For this review, take the finished solid that the model builds, in its own axes (mm). A direction names the side the tool comes from. Coordinates: 2 decimals unless noted, no trailing zeros. Loops run counter-clockwise (first coordinate to the right, second up) from the corner with the lowest first, then second, coordinate; pieces in that order, holes last. Notation, with made-up numbers: (25.25, 1.25) - (56.25, 1.25) arc R22 cw to (56.25, 29.25) - close; hole circle Ø9 at (-19.75, 85.5). An arc over 180 degrees is marked (long way). Answer as a JSON object with one key per item and string values. Group by question number.
Item 1: We need section A-A (y = 1.5). Give the boundary of the cut face in (x, z).
Item 2: We need section C-C (z = -7.5). Give the boundary of the cut face in (x, y), then the cut area to 3 significant figures.
Item 3: Clearance check with flat-ended pins moving along their axes: pin 1 (0.5 mm diameter, centred on y = 1, z = 2.5, fed in from -X); pin 2 (6 mm diameter, centred on x = 11.5, z = -9, fed in from -Y); pin 3 (3.5 mm diameter, centred on x = 10.74, z = 2, fed in from +Y); pin 4 (10 mm diameter, centred on y = 2.5, z = -9.5, fed in from +X). State where each tip first meets the part, or that it passes through.
Item 4: Mouldability with a two-part tool opening along Z and no side actions: class faces 6 (the flat face through (10, 8, -8)), 7 (the flat face through (3, 15, -14)), 8 (the cylindrical face through (6.35, 13.01, -8.08)) as released by +Z, released by -Z, zero draft, split by the parting line, or undercut.
Item 5: Tool access review of faces 1 (the cylindrical face through (1.77, 24.64, -13.1)), 2 (the flat face through (12.8, 2.5, 4.5)), 3 (the flat face through (9, 2.4, 3)), 4 (the flat face through (9, -1, -15)), 5 (the flat face through (3.5, 23, -8)): name each direction out of +Z, -Z, +X, -X, +Y, -Y from which nothing blocks a thin tool from reaching the whole face with its end or side.
Item 6: To check wall thickness, follow line 1 (Z direction, x = 10.74, y = -0.3); line 2 (Z direction, x = 10.74, y = 6.5); line 3 (X direction, y = 1, z = 2). State the ranges of each line that lie inside material, in increasing order.
Item 7: We need section B-B (y = 5.75). Give the boundary of the cut face in (x, z), then the cut area to 3 significant figures.
Item 8: We need section D-D (x = 2). Give the boundary of the cut face in (y, z), then the cut area to 3 significant figures.
from build123d import *

# Parameters (mm, degrees)
SALIENTE_EXTRUIR1_DEPTH = 10
CORTAR_EXTRUIR1_DEPTH   = 8
CROQUIS3_W              = 9
CROQUIS3_H              = 2.5
SALIENTE_EXTRUIR2_DEPTH = 5
CROQUIS4_R              = 1.5499999999999994
CORTAR_EXTRUIR2_DEPTH   = 2.5
REDONDEO1_R             = 2
CROQUIS5_R              = 2.9
CORTAR_EXTRUIR3_DEPTH   = 7.6
SALIENTE_EXTRUIR3_DEPTH = 15.5
REDONDEO2_R             = 10
REDONDEO3_R             = 3
CROQUIS8_R              = 1.5499999999999994
SALIENTE_EXTRUIR5_DEPTH = 1
CROQUIS9_W              = 5
CROQUIS9_H              = 1.700000000000001
CORTAR_EXTRUIR4_DEPTH   = 36.46565245064583


with BuildPart() as part:
    # Croquis1 → Saliente-Extruir1 (new body)
    with BuildSketch(Plane(origin=(0, 0, 0), x_dir=(1, 0, 0), z_dir=(0, 1, 0))):
        Polygon((0, 0), (18.75, 0), (18.749999999999996, 16), (-3.47e-15, 16), align=None)
    extrude(amount=SALIENTE_EXTRUIR1_DEPTH)

    # Croquis2 → Cortar-Extruir1 (cut)
    with BuildSketch(Plane.XZ):
        Polygon((0, -1.7000000000000002), (18.749999999999993, -1.6999999999999997), (18.749999999999996, -14.3), (1.51e-15, -14.3), align=None)
    extrude(amount=-CORTAR_EXTRUIR1_DEPTH, mode=Mode.SUBTRACT)

    # Croquis3 → Saliente-Extruir2 (add)
    with BuildSketch(Plane.XY):
        with Locations((10.750000000000002, 1.25)):
            Rectangle(CROQUIS3_W, CROQUIS3_H)
    extrude(amount=SALIENTE_EXTRUIR2_DEPTH)

    # Croquis4 → Cortar-Extruir2 (cut)
    with BuildSketch(Plane(origin=(0, 2.5, 0), x_dir=(1, 0, 0), z_dir=(0, 1, 0))):
        with Locations(Location((10.74, -2, 0), (0, 0, 270))):
            Circle(CROQUIS4_R)
    extrude(amount=-CORTAR_EXTRUIR2_DEPTH, mode=Mode.SUBTRACT)

    # Redondeo1
    # the kernel refuses this fillet: 2 mm, written as the material it adds along each edge
    with BuildSketch(Plane(origin=(6.25, 2.5, 0), x_dir=(-1, 0, 0), z_dir=(0, -1, 0))) as redondeo1_piece_1:
        with BuildLine():
            CenterArc((REDONDEO1_R, -REDONDEO1_R), REDONDEO1_R, 90, 90)
            Line((0, -REDONDEO1_R), (0, 0))
            Line((0, 0), (REDONDEO1_R, 0))
        make_face()
    extrude(amount=2.5)
    with BuildSketch(Plane(origin=(15.25, 0, 0), x_dir=(1, 0, 0), z_dir=(0, 1, 0))) as redondeo1_piece_2:
        with BuildLine():
            CenterArc((REDONDEO1_R, -REDONDEO1_R), REDONDEO1_R, 90, 90)
            Line((0, -REDONDEO1_R), (0, 0))
            Line((0, 0), (REDONDEO1_R, 0))
        make_face()
    extrude(amount=2.5)
    with BuildSketch(Plane(origin=(15.25, 2.5, 0), x_dir=(0, 1, 0), z_dir=(-1, 0, 0))) as redondeo1_piece_3_section:
        with BuildLine():
            CenterArc((REDONDEO1_R, -REDONDEO1_R), REDONDEO1_R, 90, 90)
            Line((0, -REDONDEO1_R), (0, 0))
            Line((0, 0), (REDONDEO1_R, 0))
        make_face()
    redondeo1_piece_3 = extrude(amount=9, mode=Mode.PRIVATE)
    redondeo1_piece_3 = redondeo1_piece_3 - Plane(origin=(10.74, 2.981912580650479, 2), x_dir=(-1.8e-16, 0, 1), z_dir=(0, 1, 0)) * Cylinder(1.5499999999999994, 26, mode=Mode.PRIVATE)
    add(redondeo1_piece_3)
    with BuildSketch(Plane(origin=(6.25, 7.5, 0), x_dir=(-1, 0, 0), z_dir=(0, -1, 0))) as redondeo1_piece_4a_section:
        with BuildLine():
            CenterArc((REDONDEO1_R, -REDONDEO1_R), REDONDEO1_R, 90, 90)
            Line((0, -REDONDEO1_R), (0, 0))
            Line((0, 0), (REDONDEO1_R, 0))
        make_face()
    redondeo1_piece_4a = extrude(amount=7.5, mode=Mode.PRIVATE)
    redondeo1_piece_4a = split(redondeo1_piece_4a, bisect_by=Plane(origin=(5.797209771466349, 2.5, 0.45279022853365075), z_dir=(0, 1, 0)), keep=Keep.TOP, mode=Mode.PRIVATE)
    with BuildSketch(Plane(origin=(15.25, 2.5, 0), x_dir=(0, 1, 0), z_dir=(-1, 0, 0))) as redondeo1_piece_4b_section:
        with BuildLine():
            CenterArc((REDONDEO1_R, -REDONDEO1_R), REDONDEO1_R, 90, 90)
            Line((0, -REDONDEO1_R), (0, 0))
            Line((0, 0), (REDONDEO1_R, 0))
        make_face()
    redondeo1_piece_4b = extrude(amount=14, mode=Mode.PRIVATE)
    redondeo1_piece_4b = split(redondeo1_piece_4b, bisect_by=Plane(origin=(6.25, 2.952790228533651, 0.45279022853365075), z_dir=(-1, 0, 0)), keep=Keep.TOP, mode=Mode.PRIVATE)
    redondeo1_piece_4 = redondeo1_piece_4a & redondeo1_piece_4b
    add(redondeo1_piece_4)
    with BuildSketch(Plane(origin=(20.25, 2.5, 0), x_dir=(0, 1, 0), z_dir=(-1, 0, 0))) as redondeo1_piece_5a_section:
        with BuildLine():
            CenterArc((REDONDEO1_R, -REDONDEO1_R), REDONDEO1_R, 90, 90)
            Line((0, -REDONDEO1_R), (0, 0))
            Line((0, 0), (REDONDEO1_R, 0))
        make_face()
    redondeo1_piece_5a = extrude(amount=14, mode=Mode.PRIVATE)
    redondeo1_piece_5a = split(redondeo1_piece_5a, bisect_by=Plane(origin=(18.75, 2.952790228533651, 0.45279022853365036), z_dir=(-1, 0, 2.2e-16)), keep=Keep.TOP, mode=Mode.PRIVATE)
    redondeo1_piece_5a = split(redondeo1_piece_5a, bisect_by=Plane(origin=(15.25, 2.952790228533651, 0.45279022853365075), z_dir=(1, 0, 0)), keep=Keep.TOP, mode=Mode.PRIVATE)
    with BuildSketch(Plane(origin=(15.25, 0, 0), x_dir=(1, 0, 0), z_dir=(0, 1, 0))) as redondeo1_piece_5b_section:
        with BuildLine():
            CenterArc((REDONDEO1_R, -REDONDEO1_R), REDONDEO1_R, 90, 90)
            Line((0, -REDONDEO1_R), (0, 0))
            Line((0, 0), (REDONDEO1_R, 0))
        make_face()
    redondeo1_piece_5b = extrude(amount=7.5, mode=Mode.PRIVATE)
    redondeo1_piece_5b = split(redondeo1_piece_5b, bisect_by=Plane(origin=(15.70279022853365, 2.5, 0.45279022853364964), z_dir=(0, 1, 0)), keep=Keep.TOP, mode=Mode.PRIVATE)
    redondeo1_piece_5 = redondeo1_piece_5a & redondeo1_piece_5b
    add(redondeo1_piece_5)
    # the kernel refuses this fillet: 2 mm, written as the material it takes off along each edge
    with BuildSketch(Plane(origin=(23.749999999999996, 10, -16), x_dir=(0, -1, 0), z_dir=(-1, 0, 0))) as redondeo1_2_piece_1:
        with BuildLine():
            CenterArc((REDONDEO1_R, REDONDEO1_R), REDONDEO1_R, 180, 90)
            Line((0, REDONDEO1_R), (0, 0))
            Line((0, 0), (REDONDEO1_R, 0))
        make_face()
    extrude(amount=28.75, mode=Mode.SUBTRACT)
    with BuildSketch(Plane(origin=(6.25, 7.5, 5), x_dir=(0, 0, -1), z_dir=(0, -1, 0))) as redondeo1_2_piece_2:
        with BuildLine():
            CenterArc((REDONDEO1_R, REDONDEO1_R), REDONDEO1_R, 180, 90)
            Line((0, REDONDEO1_R), (0, 0))
            Line((0, 0), (REDONDEO1_R, 0))
        make_face()
    extrude(amount=12.5, mode=Mode.SUBTRACT)
    with BuildSketch(Plane(origin=(15.25, -5, 5), x_dir=(0, 0, -1), z_dir=(0, 1, 0))) as redondeo1_2_piece_3:
        with BuildLine():
            CenterArc((REDONDEO1_R, REDONDEO1_R), REDONDEO1_R, 180, 90)
            Line((0, REDONDEO1_R), (0, 0))
            Line((0, 0), (REDONDEO1_R, 0))
        make_face()
    extrude(amount=12.5, mode=Mode.SUBTRACT)
    with BuildSketch(Plane(origin=(-5, 10, 0), x_dir=(0, -1, 0), z_dir=(1, 0, 0))) as redondeo1_2_piece_4:
        with BuildLine():
            CenterArc((REDONDEO1_R, REDONDEO1_R), REDONDEO1_R, 180, 90)
            Line((0, REDONDEO1_R), (0, 0))
            Line((0, 0), (REDONDEO1_R, 0))
        make_face()
    extrude(amount=28.75, mode=Mode.SUBTRACT)

    # Croquis5 → Cortar-Extruir3 (cut)
    with BuildSketch(Plane(origin=(0, 10, 0), x_dir=(1, 0, 0), z_dir=(0, 1, 0))):
        with Locations(Location((10.74, -2, 0), (0, 0, 270))):
            Circle(CROQUIS5_R)
    extrude(amount=-CORTAR_EXTRUIR3_DEPTH, mode=Mode.SUBTRACT)

    # Croquis6 → Saliente-Extruir3 (add)
    with BuildSketch(Plane(origin=(0, 10, 0), x_dir=(1, 0, 0), z_dir=(0, 1, 0))):
        Polygon((-3.04e-15, 14), (3.499999999999997, 14), (3.4999999999999982, 2), (-3.04e-15, 2), align=None)
    extrude(amount=SALIENTE_EXTRUIR3_DEPTH)

    # Redondeo2
    # the kernel refuses this fillet: 10 mm, written as the material it adds along each edge
    with BuildSketch(Plane(origin=(3.499999999999997, 10, -14), x_dir=(1, 0, -1.1e-16), z_dir=(1.1e-16, 0, 1))) as redondeo2_piece_1:
        with BuildLine():
            CenterArc((REDONDEO2_R, REDONDEO2_R), REDONDEO2_R, 180, 90)
            Line((-2.22e-15, REDONDEO2_R), (0, 0))
            Line((0, 0), (REDONDEO2_R, 0))
        make_face()
    extrude(amount=12)

    # Redondeo3
    redondeo3_edges = [part.edges().sort_by_distance(p)[0] for p in [
        (1.7499999999999976, 25.5, -2),
        (1.749999999999997, 25.5, -14),
    ]]
    fillet(redondeo3_edges, radius=REDONDEO3_R)

    # Croquis8 → Saliente-Extruir5 (add)
    # profile 1 of 2: a face of its own
    with BuildSketch(Plane.XZ):
        with BuildLine():
            Line((13.25, 5), (8.25, 5))
            ThreePointArc((8.25, 5), (6.835786437626905, 4.414213562373095), (6.25, 3.0000000000000004))
            Line((6.25, 3.0000000000000004), (6.25, 2))
            ThreePointArc((6.25, 2), (5.664213562373095, 0.5857864376269051), (4.25, 0))
            Line((4.25, 0), (-5, 1.08e-15))
            Line((-5, 1.08e-15), (-5, -1.699999999999999))
            Line((-5, -1.699999999999999), (18.749999999999993, -1.6999999999999997))
            Line((18.749999999999993, -1.6999999999999997), (18.75, 0))
            Line((18.75, 0), (17.25, 0))
            ThreePointArc((17.25, 0), (15.835786437626904, 0.5857864376269051), (15.25, 2.0000000000000004))
            Line((15.25, 2.0000000000000004), (15.25, 3))
            ThreePointArc((15.25, 3), (14.664213562373096, 4.414213562373095), (13.25, 5))
        make_face()
        with Locations(Location((10.74, 2, 0), (0, 0, 90))):
            Circle(CROQUIS8_R, mode=Mode.SUBTRACT)
    # profile 2 of 2: a face of its own
    with BuildSketch(Plane.XZ):
        Polygon((18.749999999999996, -14.3), (-5.0000000000000036, -14.299999999999999), (-5.0000000000000036, -16), (18.749999999999996, -16), align=None)
    extrude(amount=SALIENTE_EXTRUIR5_DEPTH)

    # Croquis9 → Cortar-Extruir4 (cut, through all)
    with BuildSketch(Plane(origin=(0, 0, 0), x_dir=(1, 0, 0), z_dir=(0, 1, 0))):
        with Locations((-2.5000000000000036, 15.149999999999999)):
            Rectangle(CROQUIS9_W, CROQUIS9_H)
        Polygon((-5, -1.08e-15), (0, 0), (0, 1.7000000000000002), (-5, 1.699999999999999), align=None)
    extrude(amount=-CORTAR_EXTRUIR4_DEPTH, mode=Mode.SUBTRACT)


solid = part.part
Check sheet entries:
{
 "1": {"outline": "(0, -16) - (18.75, -16) - (18.75, -14.3) - (0, -14.3) - close; (0, -1.7) - (18.75, -1.7) - (18.75, 0) - (17.25, 0) arc R2 cw to (15.25, 2) - (15.25, 3) arc R2 ccw to (13.25, 5) - (8.25, 5) arc R2 ccw to (6.25, 3) - (6.25, 2) arc R2 cw to (4.25, 0) - (0, 0) - close; hole circle Ø3.1 at (10.74, 2)"},
 "2": {"outline": "(0, 8) - (18.75, 8) - (18.75, 10) - (13.5, 10) arc R10 cw to (3.5, 20) - (3.5, 25.5) - (0, 25.5) - close", "area": "113 mm2"},
 "3": {"pin 1": "stops at x = 6.25", "pin 2": "stops at y = 8", "pin 3": "stops at y = 2.4", "pin 4": "stops at x = 18.75"},
 "4": {"face 6": "undercut", "face 7": "released by -Z", "face 8": "zero draft"},
 "5": {"face 1": "-Z, +X, -X, +Y", "face 2": "+Z, +X, -X, +Y", "face 3": "+Y", "face 4": "+Z, -Z, +X, -X, -Y", "face 5": "+Z, -Z, +X, +Y"},
 "6": {"line 1": "z = -16 to -14.3, -1.7 to 0.45, 3.55 to 5", "line 2": "z = -16 to -14.3, -1.7 to -0.9", "line 3": "x = 6.25 to 9.19, 12.29 to 15.25"},
 "7": {"outline": "(0, -16) - (18.75, -16) - (18.75, -14.3) - (0, -14.3) - close; (0, -1.7) - (18.75, -1.7) - (18.75, 0) - (12.84, 0) arc R2.9 cw to (8.64, 0) - (0, 0) - close", "area": "61.1 mm2"},
 "8": {"outline": "(-1, -16) - (8, -16) arc R2 ccw to (10, -14) - (22.5, -14) arc R3 ccw to (25.5, -11) - (25.5, -5) arc R3 ccw to (22.5, -2) - (10, -2) arc R2 ccw to (8, 0) - (-1, 0) - (-1, -1.7) - (8, -1.7) - (8, -14.3) - (-1, -14.3) - close", "area": "243 mm2"}
}
